For this review, take the finished solid that the model builds, in its own axes (mm). A direction names the side the tool comes from. Coordinates: 2 decimals unless noted, no trailing zeros. Order: outer loops, then holes, each group sorted by start corner. A loop starts at its lowest first (then second) coordinate and runs counter-clockwise, first axis right, second up.
from build123d import *

# Parameters (mm, degrees)
BOSS_EXTRUDE1_DEPTH = 22
FILLET1_R           = 0.5
SKETCH2_W           = 17.9
SKETCH2_H           = 1.4
BOSS_EXTRUDE2_DEPTH = 2


with BuildPart() as part:
    # Sketch1 → Boss-Extrude1 (new body)
    with BuildSketch(Plane.XY):
        with BuildLine():
            Line((-5.950723388, -1.667721547), (-5.452849623, -1.667721547))
            ThreePointArc((-5.452849623, -1.667721547), (-4.744239366, -1.374205568), (-4.450723388, -0.665595311))
            Line((-4.450723388, -0.665595311), (-4.450723388, 0.332278453))
            ThreePointArc((-4.450723388, 0.332278453), (-4.157207409, 1.04088871), (-3.448597153, 1.334404689))
            Line((-3.448597153, 1.334404689), (-2.452849623, 1.334404689))
            ThreePointArc((-2.452849623, 1.334404689), (-1.744239366, 1.04088871), (-1.450723388, 0.332278453))
            Line((-1.450723388, 0.332278453), (-1.450723388, -4.165595311))
            ThreePointArc((-1.450723388, -4.165595311), (-1.744239366, -4.874205568), (-2.452849623, -5.167721547))
            Line((-2.452849623, -5.167721547), (-5.950723388, -5.167721547))
            Line((-5.950723388, -5.167721547), (-5.950723388, -1.667721547))
        make_face()
    extrude(amount=BOSS_EXTRUDE1_DEPTH)

    # Fillet1
    fillet1_edges = [part.edges().sort_by_distance(p)[0] for p in [
        (-1.744239366, 1.04088871, 22),
        (-5.701786505, -1.667721547, 0),
        (-4.744239366, -1.374205568, 0),
        (-4.450723388, -0.166658429, 0),
        (-4.157207409, 1.04088871, 0),
        (-2.950723388, 1.334404689, 0),
        (-1.744239366, 1.04088871, 0),
        (-1.450723388, -1.916658429, 0),
        (-1.744239366, -4.874205568, 0),
        (-2.950723388, 1.334404689, 22),
        (-4.157207409, 1.04088871, 22),
        (-4.450723388, -0.166658429, 22),
        (-4.744239366, -1.374205568, 22),
        (-5.701786505, -1.667721547, 22),
        (-4.201786505, -5.167721547, 22),
        (-1.744239366, -4.874205568, 22),
        (-1.450723388, -1.916658429, 22),
        (-4.201786505, -5.167721547, 0),
    ]]
    fillet(fillet1_edges, radius=FILLET1_R)

    # Sketch2 → Boss-Extrude2 (add)
    with BuildSketch(Plane.ZY.offset(5.950723388)):
        with Locations((11, -3.417721547)):
            Rectangle(SKETCH2_W, SKETCH2_H)
    extrude(amount=BOSS_EXTRUDE2_DEPTH)


solid = part.part
1. Take a section at B-B, the plane z = 20.5. Give the boundary of the cut face in (x, y), plus the area to 3 significant figures.
Answer below:
outline: (-5.95, -5.17) - (-2.45, -5.17) arc R1 ccw to (-1.45, -4.17) - (-1.45, 0.33) arc R1 ccw to (-2.45, 1.33) - (-3.45, 1.33) arc R1 ccw to (-4.45, 0.33) - (-4.45, -0.67) arc R1 cw to (-5.45, -1.67) - (-5.95, -1.67) - close
area: 24.3 mm2
2. Take a section at D-D, the plane z = 8.5. Give the boundary of the cut face in (x, y), plus the area to 3 significant figures.
Answer below:
outline: (-7.95, -4.12) - (-5.95, -4.12) - (-5.95, -5.17) - (-2.45, -5.17) arc R1 ccw to (-1.45, -4.17) - (-1.45, 0.33) arc R1 ccw to (-2.45, 1.33) - (-3.45, 1.33) arc R1 ccw to (-4.45, 0.33) - (-4.45, -0.67) arc R1 cw to (-5.45, -1.67) - (-5.95, -1.67) - (-5.95, -2.72) - (-7.95, -2.72) - close
area: 27.1 mm2
3. Machinability: for faces 4 (the face through (-7, -3, 19.95)), 5 (the face through (-3, -2, 22)), 6 (the face through (-4.451, 0, 11)), 7 (the face through (-7, -3, 2.05)), which of the approach directions +Z, -Z, +X, -X, +Y, -Y give a long, thin tool a straight path to every point of the face, cutting with its end or side? Answer none if there is none.
Answer below:
face 4: +Z, -X, +Y, -Y
face 5: +Z, +X, -X, +Y, -Y
face 6: +Z, -Z, -X, +Y
face 7: -Z, -X, +Y, -Y
4. The part is to be moulded in two halves that separate along Y. For faces 1 (the face through (-4.165, 1.033, 10.853)), 2 (the face through (-7.951, -3, 11)), 3 (the face through (-7, -4.118, 11)), say which applies: +Y half, -Y half, draft (parallel to the pull), parting line (faces both ways), or undercut.
Answer below:
face 1: +Y half
face 2: draft
face 3: -Y half
5. Take a section at A-A, the plane y = -3.5. Give the boundary of the cut face in (x, z), plus the area to 3 significant figures.
Answer below:
outline: (-7.95, 2.05) - (-5.95, 2.05) - (-5.95, 0) - (-1.95, 0) arc R0.5 ccw to (-1.45, 0.5) - (-1.45, 21.5) arc R0.5 ccw to (-1.95, 22) - (-5.95, 22) - (-5.95, 19.95) - (-7.95, 19.95) - close
area: 135 mm2
6. Take a section at C-C, the plane x = -6.5. Give the boundary of the cut face in (y, z), plus the area to 3 significant figures.
Answer below:
outline: (-4.12, 2.05) - (-2.72, 2.05) - (-2.72, 19.95) - (-4.12, 19.95) - close
area: 25.1 mm2
7. Clearance check with flat-ended pins moving along their axes: pin 1 Ø1.1 at (x, y) = (-7.5, -3) entering from +Z; pin 2 Ø2 at (x, z) = (-7.5, 10) entering from +Y; pin 3 Ø1 at (x, z) = (-6, 20) entering from +Y. State where each tip first meets the part, or that it passes through.
Answer below:
pin 1: stops at z = 19.95
pin 2: stops at y = -2.72
pin 3: stops at y = -1.67
8. To check wall thickness, follow L1, parallel to Y at x = -7.25, z = 12.5; L2, parallel to X at y = -2, z = 6; L3, parallel to Y at x = -3.5, z = 19.25. State the ranges of each line that lie inside material, in increasing order.
Answer below:
L1: y = -4.12 to -2.72
L2: x = -5.95 to -1.45
L3: y = -5.17 to 1.33
